```python
from build123d import *

# Parameters (mm, degrees)
SKETCH1_W           = 38
SKETCH1_H           = 36
BOSS_EXTRUDE1_DEPTH = 26
SKETCH2_W           = 19
SKETCH2_H           = 32.5
CUT_EXTRUDE1_DEPTH  = 54.935146241
CUT_EXTRUDE2_REACH  = 60.447
CUT_EXTRUDE3_REACH  = 60.447
FILLET1_R           = 1
FILLET2_R           = 3.5
FILLET3_R           = 5


with BuildPart() as part:
    # Sketch1 → Boss-Extrude1 (new body)
    with BuildSketch(Plane.XY.offset(13)):
        with Locations((19, 18)):
            Rectangle(SKETCH1_W, SKETCH1_H)
    extrude(amount=-BOSS_EXTRUDE1_DEPTH)

    # Sketch2 → Cut-Extrude1 (cut, through all)
    with BuildSketch(Plane(origin=(38, 0, 0), x_dir=(0, 0, -1), z_dir=(1, 0, 0))):
        with Locations((0, 19.75)):
            Rectangle(SKETCH2_W, SKETCH2_H)
    extrude(amount=-CUT_EXTRUDE1_DEPTH, mode=Mode.SUBTRACT)

    # Sketch3 → Cut-Extrude2 (cut, up to next)
    with BuildSketch(Plane.XY.offset(13), mode=Mode.PRIVATE) as cut_extrude2_sk1:
        with BuildLine():
            Line((22.5, 36), (0, 36))
            Line((0, 36), (0, 8.734288837))
            Line((0, 8.734288837), (24.385099457, 22.083618886))
            ThreePointArc((24.385099457, 22.083618886), (26.303250734, 26.500012997), (22.5, 29.45282947))
            ThreePointArc((22.5, 29.45282947), (19.226414735, 32.726414735), (22.5, 36))
        make_face()
    cut_extrude2_tool1 = extrude(cut_extrude2_sk1.sketch, amount=-CUT_EXTRUDE2_REACH, mode=Mode.PRIVATE) & part.part
    add(cut_extrude2_tool1.solids().sort_by_distance((10.485992, 24.898976, 13))[0], mode=Mode.SUBTRACT)

    # Sketch4 → Cut-Extrude3 (cut, up to next)
    with BuildSketch(Plane(origin=(0, 0, -13), x_dir=(-1, 0, 0), z_dir=(0, 0, -1)), mode=Mode.PRIVATE) as cut_extrude3_sk1:
        with BuildLine():
            Line((-23.85253982, 21.972620507), (0, 10.7))
            Line((0, 10.7), (0, 36))
            Line((0, 36), (-22.5, 36))
            ThreePointArc((-22.5, 36), (-18.5, 32), (-22.5, 28))
            ThreePointArc((-22.5, 28), (-25.588635116, 25.527643349), (-23.85253982, 21.972620507))
        make_face()
    cut_extrude3_tool1 = extrude(cut_extrude3_sk1.sketch, amount=-CUT_EXTRUDE3_REACH, mode=Mode.PRIVATE) & part.part
    add(cut_extrude3_tool1.solids().sort_by_distance((10.140401, 25.382196, -13))[0], mode=Mode.SUBTRACT)

    # Fillet1
    fillet1_edges = [part.edges().sort_by_distance(p)[0] for p in [
        (19, 3.5, -9.5),
        (19, 3.5, 9.5),
    ]]
    fillet(fillet1_edges, radius=FILLET1_R)

    # Fillet2
    fillet2_edges = [part.edges().sort_by_distance(p)[0] for p in [
        (19, 0, -13),
        (19, 0, 13),
    ]]
    fillet(fillet2_edges, radius=FILLET2_R)

    # Fillet3
    fillet3_edges = [part.edges().sort_by_distance(p)[0] for p in [
        (38, 36, 11.25),
        (38, 36, -11.25),
    ]]
    fillet(fillet3_edges, radius=FILLET3_R)


solid = part.part
```
CAD build for the part. Positions are in the model's coordinates, mm. A direction names the side the tool comes from. Round coordinates to 2 decimals unless told otherwise and drop trailing zeros. Write each loop counter-clockwise with the first axis right and the second up, starting at its lowest first coordinate (ties: lowest second). Pieces come first, ordered by that corner, then holes.
Item 1: Tool access for faces 4 (the flat face through (19, 3.5, 0)), 5 (the flat face through (0, 3, 0)), 6 (the cylindrical face through (19.27, 1, -11.95)), 7 (the flat face through (12.093, 16.415, -11.274)), 8 (the cylindrical face through (19.227, 32.654, 11.274)): list every direction of +Z, -Z, +X, -X, +Y, -Y with a clear straight run to the whole face (end or side of a thin tool).
Filled in:
face 4: +X, -X, +Y
face 5: +Z, -Z, -X, +Y, -Y
face 6: -Z, +X, -X, -Y
face 7: +Z, -Z, -X
face 8: +Z, -X
Item 2: Drop a flat-ended pin along its axis: pin 1 Ø5 at (x, z) = (23, -3) entering from +Y. Give the stop position or say it passes through.
Filled in:
pin 1: stops at y = 3.5
Item 3: Band-saw the part on B-B on x = 6.5. Write the cut outline in (y, z), then the cut area to 3 significant figures.
Filled in:
outline: (0, -9.5) arc R3.5 ccw to (3.5, -13) - (13.77, -13) - (13.77, -9.5) - (4.5, -9.5) arc R1 cw to (3.5, -8.5) - (3.5, 8.5) arc R1 cw to (4.5, 9.5) - (12.29, 9.5) - (12.29, 13) - (3.5, 13) arc R3.5 ccw to (0, 9.5) - close
area: 153 mm2
Item 4: Mould opens along Z. For faces 1 (the cylindrical face through (19.27, 1.05, 12)), 2 (the cylindrical face through (18.5, 32.1, -11.3)), 3 (the flat face through (23, 17, -9.5)) say: released by +Z, released by -Z, zero draft, split by the parting line, or undercut.
Filled in:
face 1: released by +Z
face 2: zero draft
face 3: undercut
Item 5: Band-saw the part on C-C on z = -7.75. Write the cut outline in (x, y), then the cut area to 3 significant figures.
Filled in:
outline: (0, 0) - (38, 0) - (38, 3.5) - (0, 3.5) - close
area: 133 mm2
Item 6: Band-saw the part on D-D on y = 26.5. Write the cut outline in (x, z), then the cut area to 3 significant figures.
Filled in:
outline: (25.19, -13) - (38, -13) - (38, -9.5) - (25.19, -9.5) - close; (26.3, 9.5) - (38, 9.5) - (38, 13) - (26.3, 13) - close
area: 85.8 mm2
Item 7: Drill centre lines: L1, parallel to Z at x = 28.5, y = 24.5; L2, parallel to Y at x = 10, z = 6.75; L3, parallel to Y at x = 13, z = 10. Where is each one in solid material? Low to high.
Filled in:
L1: z = -13 to -9.5, 9.5 to 13
L2: y = 0 to 3.5
L3: y = 0.04 to 15.85
Item 8: Band-saw the part on A-A on y = 19.5. Write the cut outline in (x, z), then the cut area to 3 significant figures.
Filled in:
outline: (18.62, -13) - (38, -13) - (38, -9.5) - (18.62, -9.5) - close; (19.67, 9.5) - (38, 9.5) - (38, 13) - (19.67, 13) - close
area: 132 mm2
